Input: part model. Units: mm. Frame: model coordinates. A direction names the side the tool comes from. Give positions to 0.01 mm unless a question says otherwise; leave off trailing zeros. Loops run counter-clockwise (first coordinate to the right, second up) from the corner with the lowest first, then second, coordinate; pieces in that order, holes last. Notation, with made-up numbers: M 20.5,27.5 L 44.5,27.5 A18 cw 44.5,54.5 Z; hole C 15.25,-3 d1. An arc over 180 degrees is marked long. One line per item, written item: value. Start each with the question number.
(1) Section B-B on x = 42. Output: boundary loops of the cut face in (y, z), plus the area to 3 significant figures.
(2) Access query for faces 1 (the flat face through (0, 27, -9)), 2 (the flat face through (-1, 21, -7)). Directions: +Z, -Z, +X, -X, +Y, -Y. A direction counts if a zero-diameter tool reaches every point of the face in a straight line with its end or side. Return the directions, or none.
(3) Section A-A on y = -32. Output: boundary loops of the cut face in (x, z), plus the area to 3 significant figures.
(4) Ray query, line 1 along Y through (x, z) = (-42, -9); line 2 along Y through (x, z) = (-2, -10.4); line 3 along X through (y, z) = (72, -8.65). Return the intervals inside material, ascending. Write a range as from..to.
(5) Section C-C on z = -8.75. Output: boundary loops of the cut face in (x, y), plus the area to 3 significant figures.
(6) Pin query (flat end, axial travel): P1, Ø11, axis at x = -1, y = 40.5, coming from the +Z side; P2, Ø3, axis at x = -42, y = 72, coming from the +Z side. Return the tip coordinate at first contact, or that it passes through.
(7) Pull-direction query (Y, two-part tool) for faces 3 (the cylindrical face through (42.968, -30.482, -8.774)), 4 (the flat face through (-50, 19, -10)), 5 (the flat face through (-1, 80, -10)); classes: released by +Y, released by -Y, zero draft, split by the parting line, or undercut.
(8) Section D-D on x = -8. Output: boundary loops of the cut face in (y, z).
```python
from build123d import *

# Parameters (mm, degrees)
BOX041_W          = 41
BOX041_H          = 22
BOX041_DEPTH      = 10
CYLINDER018_R     = 1.8
CYLINDER018_DEPTH = 6.6
ARRAY016_X_COUNT  = 2
ARRAY016_X_PITCH  = 84
ARRAY016_Y_COUNT  = 2
ARRAY016_Y_PITCH  = 104
BOX042_W          = 41
BOX042_H          = 22
BOX042_DEPTH      = 10
BOX040_W          = 100
BOX040_H          = 120
BOX040_DEPTH      = 5
FILLET008_R       = 1


with BuildPart() as obj1:
    # Box041 → Box041 (new body)
    with BuildSketch(Plane(origin=(-20.5, -9, -11), x_dir=(1, 0, 0), z_dir=(0, 0, 1))):
        with Locations((20.5, 11)):
            Rectangle(BOX041_W, BOX041_H)
    extrude(amount=BOX041_DEPTH)


with BuildPart() as cone:
    # Cone → Cone (revolve)
    with BuildSketch(Plane.XZ):
        Polygon((0, 0), (2.6, 0), (1.8, 1.5), (0, 1.5), align=None)
    revolve(axis=Axis((0, 0, 0), (0, 0, 1)))


with BuildPart() as magnet_stand_cube_hole_array_clone:
    # Cylinder018 → Cylinder018 (new body)
    with BuildSketch(Plane.XY):
        Circle(CYLINDER018_R)
    extrude(amount=CYLINDER018_DEPTH)

    # Fusion005004012: union Cone
    add(cone.part)

    # Array016 X: magnet stand cube hole array clone ×2


with BuildPart() as magnet_stand_cube_hole_array_clone_1:
    add(magnet_stand_cube_hole_array_clone.part)
    with Locations(*[(i * ARRAY016_X_PITCH, 0, 0) for i in range(1, ARRAY016_X_COUNT)]):
        add(magnet_stand_cube_hole_array_clone.part)

    # Array016 Y: magnet stand cube hole array clone ×2


with BuildPart() as magnet_stand_cube_hole_array_clone_2:
    add(magnet_stand_cube_hole_array_clone_1.part)
    with Locations(*[(0, i * ARRAY016_Y_PITCH, 0) for i in range(1, ARRAY016_Y_COUNT)]):
        add(magnet_stand_cube_hole_array_clone_1.part)


with BuildPart() as magnet_stand_cube_hole_array_clone_3:
    # Array016 placement: moved
    add(magnet_stand_cube_hole_array_clone_2.part.moved(Location((-42, -32, -12))))


with BuildPart() as obj2:
    # Box042 → Box042 (new body)
    with BuildSketch(Plane(origin=(-20.5, 27, -11), x_dir=(1, 0, 0), z_dir=(0, 0, 1))):
        with Locations((20.5, 11)):
            Rectangle(BOX042_W, BOX042_H)
    extrude(amount=BOX042_DEPTH)

    # Fusion005004011: union obj1, magnet stand cube hole array clone
    add(obj1.part)
    add(magnet_stand_cube_hole_array_clone_3.part)


with BuildPart() as obj3:
    # Box040 → Box040 (new body)
    with BuildSketch(Plane(origin=(-50, -40, -12), x_dir=(1, 0, 0), z_dir=(0, 0, 1))):
        with Locations((50, 60)):
            Rectangle(BOX040_W, BOX040_H)
    extrude(amount=BOX040_DEPTH)

    # Fillet008
    fillet008_edges = [obj3.edges().sort_by_distance(p)[0] for p in [
        (-50, -40, -9.5),
        (-50, 80, -9.5),
        (50, -40, -9.5),
        (50, 80, -9.5),
    ]]
    fillet(fillet008_edges, radius=FILLET008_R)

    # Cut002003010: cut obj2
    add(obj2.part, mode=Mode.SUBTRACT)


solid = obj3.part
```
Output values:
1. outline: M -40,-12 L -34.6,-12 L -33.8,-10.5 L -33.8,-7 L -40,-7 Z; M -30.2,-10.5 L -29.4,-12 L 69.4,-12 L 70.2,-10.5 L 70.2,-7 L -30.2,-7 Z; M 73.8,-10.5 L 74.6,-12 L 80,-12 L 80,-7 L 73.8,-7 Z
1. area: 562 mm²
2. face 1: +Z
2. face 2: +Z, +X, -X, +Y, -Y
3. outline: M -50,-12 L -44.6,-12 L -43.8,-10.5 L -43.8,-7 L -50,-7 Z; M -40.2,-10.5 L -39.4,-12 L 39.4,-12 L 40.2,-10.5 L 40.2,-7 L -40.2,-7 Z; M 43.8,-10.5 L 44.6,-12 L 50,-12 L 50,-7 L 43.8,-7 Z
3. area: 462 mm²
4. line 1: y = -40..-33.8, -30.2..70.2, 73.8..80
4. line 2: y = -40..-9, 13..27, 49..80
4. line 3: x = -50..-43.8, -40.2..40.2, 43.8..50
5. outline: M -50,-39 A1 ccw -49,-40 L 49,-40 A1 ccw 50,-39 L 50,79 A1 ccw 49,80 L -49,80 A1 ccw -50,79 Z; hole C -42,-32 d3.6; hole C -42,72 d3.6; hole M -20.5,-9 L 20.5,-9 L 20.5,13 L -20.5,13 Z; hole M -20.5,27 L 20.5,27 L 20.5,49 L -20.5,49 Z; hole C 42,-32 d3.6; hole C 42,72 d3.6
5. area: 10,200 mm²
6. P1: stops at z = -11
6. P2: passes through
7. face 3: undercut
7. face 4: zero draft
7. face 5: released by +Y
8. outline: M -40,-12 L 80,-12 L 80,-7 L 49,-7 L 49,-11 L 27,-11 L 27,-7 L 13,-7 L 13,-11 L -9,-11 L -9,-7 L -40,-7 Z
